Read the model definition and answer for the solid it produces. Units are mm, in the model's axes. A direction names the side the tool comes from. Round coordinates to 2 decimals unless told otherwise and drop trailing zeros. Loops run counter-clockwise (first coordinate to the right, second up) from the corner with the lowest first, then second, coordinate; pieces in that order, holes last. Notation, with made-up numbers: (9, 68.25) - (15, 68.25) arc R11 ccw to (15, 73.25) - close; hole circle Ø6 at (-11, 20). An arc over 180 degrees is marked (long way). Answer as CSV lines item,"result".
Autodesk Fusion 360 part; units mm, degrees
sketch "スケッチ1" plane through (0, 0, 0) normal (1, 0, 0) x (0, 0, -1)
  line L0 (0, 2) -> (0, 0)
  line L1 (3, 0) -> (24, 0)
  line L2 (27, 0) -> (27, 2)
  line L3 (27, 2) -> (18, 2)
  line L4 (18, 2) -> (13, 7)
  line L5 (13, 7) -> (13, 12)
  line L6 (13, 12) -> (11, 12)
  line L7 (11, 12) -> (11, 6)
  line L8 (7, 2) -> (0, 2)
  line L9 (11, 6) -> (7, 2)
  line L10 (3, 0) -> (3, -3)
  line L11 (3, -3) -> (0, -3)
  line L12 (0, -3) -> (0, 0)
  line L13 (24, 0) -> (24, -3)
  line L14 (24, -3) -> (27, -3)
  line L15 (27, -3) -> (27, 0)
  point P0 (11, 2)
  dimension "d1" = 4
  dimension "d2" = 4
  dimension "d15" = 27
  dimension "d16" = 3
  dimension "d17" = 3
  dimension "d18" = 3
  dimension "d19" = 3
extrude "押し出し1" add sketch "スケッチ1" along normal blind 33
chamfer "面取り1" distance 0.5 angle 45 1 edges at (0, -0.5, -27)
chamfer "面取り2" distance 0.5 angle 45 1 edges at (0, -0.5, 0)
chamfer "面取り3" distance 0.5 angle 45 1 edges at (33, -0.5, -27)
chamfer "面取り4" distance 0.5 angle 45 1 edges at (33, -0.5, 0)
1) A cutting plane is placed at A-A, the plane y = -1.75. Determine the outline of the cut face in (x, z), plus the area to 4 significant figures.
Entries:
outline,"(0, -26.5) - (0.5, -27) - (32.5, -27) - (33, -26.5) - (33, -24) - (0, -24) - close; (0, -3) - (33, -3) - (33, -0.5) - (32.5, 0) - (0.5, 0) - (0, -0.5) - close"
area,"197.5 mm^2"
2) The mould has two halves that part along Z. Classify faces 5 (the face through (16, -1, -27)), 6 (the face through (16, -3, -25)), 7 (the face through (16, 9, -11)), 8 (the face through (16, -1, -3)): pulls with the +Z half, pulls with the -Z half, needs draft (parallel to the pull), parting line crosses it, or undercut.
Entries:
face 5,"pulls with the -Z half"
face 6,"needs draft"
face 7,"pulls with the +Z half"
face 8,"undercut"
3) A tool of negligible diameter and unlimited length cuts with its end or side. For faces 1 (the face through (16, 0, -13)), 2 (the face through (16, 2, -23)), 3 (the face through (16, 12, -12)), 4 (the face through (16, 2, -4)), from which of +Z, -Z, +X, -X, +Y, -Y can it reach the whole face along a straight path? Write none if from no direction.
Entries:
face 1,"+X, -X, -Y"
face 2,"-Z, +X, -X, +Y"
face 3,"+Z, -Z, +X, -X, +Y"
face 4,"+Z, +X, -X, +Y"
4) Each of these flat-tipped pins is pushed along its axis until it touches: P1, Ø2, axis at x = 14.5, z = -2.5, coming from the +Y side; P2, Ø3.5, axis at x = 18, y = -1.5, coming from the +Z side; P3, Ø2, axis at x = 10, y = 6.5, coming from the -Z side; P4, Ø6.5, axis at x = 22.5, z = -18.5, coming from the -Y side. Where does it stop, or does it pass through?
Entries:
P1,"stops at y = 2"
P2,"stops at z = 0"
P3,"stops at z = -14.5"
P4,"stops at y = 0"
5) A cutting plane is placed at D-D, the plane y = 5. Determine the outline of the cut face in (x, z), plus the area to 3 significant figures.
Entries:
outline,"(0, -15) - (33, -15) - (33, -10) - (0, -10) - close"
area,"165 mm^2"
6) Find the intervals of material crossed by line 1 (Z direction, x = 20.5, y = -2.5); line 2 (Y direction, x = 31.5, z = -25); line 3 (Y direction, x = 27, z = -5.5), in increasing order.
Entries:
line 1,"z = -27 to -24, -3 to 0"
line 2,"y = -3 to 2"
line 3,"y = 0 to 2"
7) A cutting plane is placed at C-C, the plane z = -21. Determine the outline of the cut face in (x, y), plus the area to 3 significant figures.
Entries:
outline,"(0, 0) - (33, 0) - (33, 2) - (0, 2) - close"
area,"66.0 mm^2"
8) A cutting plane is placed at B-B, the plane x = 9.5. Determine the outline of the cut face in (y, z), plus the area to 4 significant figures.
Entries:
outline,"(-3, -27) - (2, -27) - (2, -18) - (7, -13) - (12, -13) - (12, -11) - (6, -11) - (2, -7) - (2, 0) - (-3, 0) - (-3, -3) - (0, -3) - (0, -24) - (-3, -24) - close"
area,"112.5 mm^2"
